Design review of the part built by this model. Coordinates are the model's own, in mm. A direction names the side the tool comes from. Give positions to 0.01 mm unless a question says otherwise; leave off trailing zeros. Answer in a Markdown table with one row per item. Add a question column.
```python
from build123d import *

# Parameters (mm, degrees)
SKETCH1_W           = 182
SKETCH1_H           = 78
BOSS_EXTRUDE1_DEPTH = 170
SKETCH3_R           = 2.5
CUT_EXTRUDE1_DEPTH  = 5
SKETCH4_W           = 40
SKETCH4_H           = 26
CUT_EXTRUDE2_DEPTH  = 3.5
FILLET1_R           = 4


with BuildPart() as part:
    # Sketch1 → Boss-Extrude1 (new body)
    with BuildSketch(Plane(origin=(0, 0, 0), x_dir=(1, 0, 0), z_dir=(0, 1, 0))):
        Rectangle(SKETCH1_W, SKETCH1_H)
    extrude(amount=BOSS_EXTRUDE1_DEPTH)

    # Sketch3 → Cut-Extrude1 (cut)
    with BuildSketch(Plane(origin=(0, 170, 0), x_dir=(1, 0, 0), z_dir=(0, 1, 0))):
        with Locations(Location((63, -28, 0), (0, 0, 270))):
            Circle(SKETCH3_R)
        with Locations(Location((-63, -28, 0), (0, 0, 90))):
            Circle(SKETCH3_R)
    extrude(amount=-CUT_EXTRUDE1_DEPTH, mode=Mode.SUBTRACT)

    # Sketch4 → Cut-Extrude2 (cut)
    with BuildSketch(Plane(origin=(0, 170, 0), x_dir=(1, 0, 0), z_dir=(0, 1, 0))):
        with Locations((-71, -26)):
            Rectangle(SKETCH4_W, SKETCH4_H)
        with Locations((71, -26)):
            Rectangle(SKETCH4_W, SKETCH4_H)
    extrude(amount=-CUT_EXTRUDE2_DEPTH, mode=Mode.SUBTRACT)

    # Fillet1
    fillet1_edges = [part.edges().sort_by_distance(p)[0] for p in [
        (-51, 168.25, 13),
        (51, 168.25, 13),
    ]]
    fillet(fillet1_edges, radius=FILLET1_R)


solid = part.part
```
1) Machinability: for faces 5 (the face through (-52.203, 168.226, 14.141)), 6 (the face through (-63.1, 165.8, 30.5)), 7 (the face through (-91, 84, 1)), 8 (the face through (52.203, 168.226, 14.141)), 9 (the face through (-1, 84, 39)), which of the approach directions +Z, -Z, +X, -X, +Y, -Y give a long, thin tool a straight path to every point of the face, cutting with its end or side? Answer none if there is none.
2) Mouldability with a two-part tool opening along Z and no side actions: class faces 1 (the face through (63.1, 165.8, 25.5)), 2 (the face through (-63, 165, 28)), 3 (the face through (-1, 84, -39)), 4 (the face through (71, 166.5, 26)) as +Z half, -Z half, draft (parallel to the pull), parting line (faces both ways), or undercut.
3) For L1, parallel to X at y = 166, z = 28; L2, parallel to Y at x = -77.5, z = 24, list the stretches that pass through material, from the lowest coordinate up.
4) Clearance check with flat-ended pins moving along their axes: P1, Ø8, axis at x = -66, z = 23.5, coming from the +Y side; P2, Ø2.5, axis at x = -63.5, z = 28.5, coming from the +Y side; P3, Ø1.8, axis at x = -78, y = 169, coming from the +Z side; P4, Ø2, axis at x = 32.5, z = -25, coming from the -Y side. State where each tip first meets the part, or that it passes through.
Verdict:
| question | item | result |
|---|---|---|
| 1 | face 5 | +Z, -X, +Y |
| 1 | face 6 | +Y |
| 1 | face 7 | +Z, -Z, -X, +Y, -Y |
| 1 | face 8 | +Z, +X, +Y |
| 1 | face 9 | +Z, +X, -X, +Y, -Y |
| 2 | face 1 | undercut |
| 2 | face 2 | undercut |
| 2 | face 3 | -Z half |
| 2 | face 4 | draft |
| 3 | L1 | x = -91 to -65.5, -60.5 to 60.5, 65.5 to 91 |
| 3 | L2 | y = 0 to 166.5 |
| 4 | P1 | stops at y = 166.5 |
| 4 | P2 | stops at y = 165 |
| 4 | P3 | stops at z = 13 |
| 4 | P4 | stops at y = 0 |
